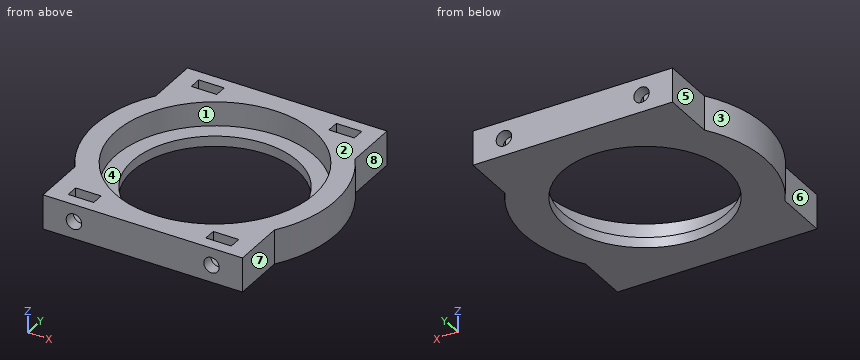
from build123d import *

# Parameters (mm, degrees)
CROQUIS1_R              = 28.9
SALIENTE_EXTRUIR1_DEPTH = 5
CROQUIS2_R              = 28.9
CROQUIS2_R_2            = 24
SALIENTE_EXTRUIR2_DEPTH = 3
CORTAR_EXTRUIR1_DEPTH   = 3.6
CROQUIS6_R              = 2.25
CORTAR_EXTRUIR2_DEPTH   = 10


with BuildPart() as part:
    # Croquis1 → Saliente-Extruir1 (new, symmetric)
    with BuildSketch(Plane.XY):
        with BuildLine():
            Line((-29, 19.595917942), (-29, 35))
            Line((-29, 35), (29, 35))
            Line((29, 35), (29, 19.595917942))
            ThreePointArc((29, 19.595917942), (35, 0), (29, -19.595917942))
            Line((29, -19.595917942), (29, -35))
            Line((29, -35), (-29, -35))
            Line((-29, -35), (-29, -19.595917942))
            ThreePointArc((-29, -19.595917942), (-35, 0), (-29, 19.595917942))
        make_face()
        Circle(CROQUIS1_R, mode=Mode.SUBTRACT)
    extrude(amount=SALIENTE_EXTRUIR1_DEPTH, both=True)

    # Croquis2 → Saliente-Extruir2 (add)
    with BuildSketch(Plane(origin=(0, 0, -5), x_dir=(-1, 0, 0), z_dir=(0, 0, -1))):
        Circle(CROQUIS2_R)
        Circle(CROQUIS2_R_2, mode=Mode.SUBTRACT)
    extrude(amount=-SALIENTE_EXTRUIR2_DEPTH)

    # Croquis5 → Cortar-Extruir1 (cut)
    with BuildSketch(Plane(origin=(0, 28, 0), x_dir=(1, 0, 0), z_dir=(0, 1, 0))):
        Polygon((-23.7, -2.136195996), (-23.7, -5), (-16.3, -5), (-16.3, -2.136195996), (-16.3, 2.136195996), (-20, 4.272391992), (-23.7, 2.136195996), align=None)
        Polygon((16.3, 2.136195996), (16.3, -2.136195996), (16.3, -5), (23.7, -5), (23.7, -2.136195996), (23.7, 2.136195996), (20, 4.272391992), align=None)
    cortar_extruir1 = extrude(amount=CORTAR_EXTRUIR1_DEPTH, mode=Mode.SUBTRACT)

    # Croquis6 → Cortar-Extruir2 (cut)
    with BuildSketch(Plane(origin=(0, 35, 0), x_dir=(1, 0, 0), z_dir=(0, 1, 0))):
        with Locations(Location((-20, 0, 0), (0, 0, 270))):
            Circle(CROQUIS6_R)
        with Locations(Location((20, 0, 0), (0, 0, 270))):
            Circle(CROQUIS6_R)
    cortar_extruir2 = extrude(amount=-CORTAR_EXTRUIR2_DEPTH, mode=Mode.SUBTRACT)

    # Simetría1: Cortar-Extruir1, Cortar-Extruir2 across plane
    add(cortar_extruir1.mirror(Plane.ZX), mode=Mode.SUBTRACT)
    add(cortar_extruir2.mirror(Plane.ZX), mode=Mode.SUBTRACT)


solid = part.part
Check sheet for the modelled part. Datum: model origin and axes. Units: mm. Face numbers are marked on the shaded views. A direction names the side the tool comes from. Give positions to 0.01 mm unless a question says otherwise; leave off trailing zeros. Loops run counter-clockwise (first coordinate to the right, second up) from the corner with the lowest first, then second, coordinate; pieces in that order, holes last. Notation, with made-up numbers: M 19.25,85.25 L 49.25,85.25 A24 ccw 49.25,100.25 Z; hole C 68.5,-20.75 d10. An arc over 180 degrees is marked long. Use a Markdown table: item, result. Add a question column.
Q1. Sectioned sample at C-C, the plane z = -3.25. Record the cut outline in (x, y), then the cut area to 3 significant figures.
Q2. Sectioned sample at A-A, the plane y = 0. Record the cut outline in (x, z).
Q3. Go/stop test with flat-tipped pins: pin 1 (3 mm diameter, centred on y = -30.5, z = 0.5, fed in from +X); pin 2 (4 mm diameter, centred on x = 20, z = 0, fed in from +Y); pin 3 (1.1 mm diameter, centred on y = -30.5, z = 2, fed in from -X); pin 4 (8 mm diameter, centred on x = 7.5, y = 16.5, fed in from -Z). Record where each tip stops, or that it passes through.
Q4. Tool access check on the marked faces 5, 6, 7 and 8. Record the directions out of +Z, -Z, +X, -X, +Y, -Y that give a thin tool (end or side, any length) a straight path to the whole face; none if there is none.
Q5. Mould release check, pull along Y, two halves, no side actions. Record for the marked faces 1, 2, 3 and 4: pulls with the +Y half, pulls with the -Y half, needs draft (parallel to the pull), parting line crosses it, or undercut.
Q6. Scan lines: line 1 along X through (y, z) = (-0.5, 1.75); line 2 along Z through (x, y) = (-20, -27). Record each from-to range of solid material in increasing order. Write a range as [from, to].
Verdict:
| question | item | result |
|---|---|---|
| 1 | outline | M -29,-35 L 29,-35 L 29,-19.6 A35 ccw 29,19.6 L 29,35 L -29,35 L -29,19.6 A35 ccw -29,-19.6 Z; hole C 0,0 d48; hole M -21.77,-31.6 L -18.23,-31.6 L -18.23,-28 L -21.77,-28 Z; hole M -21.77,28 L -18.23,28 L -18.23,31.6 L -21.77,31.6 Z; hole M 18.23,-31.6 L 21.77,-31.6 L 21.77,-28 L 18.23,-28 Z; hole M 18.23,28 L 21.77,28 L 21.77,31.6 L 18.23,31.6 Z |
| 1 | area | 2,520 mm^2 |
| 2 | outline | M -35,-5 L -24,-5 L -24,-2 L -28.9,-2 L -28.9,5 L -35,5 Z; M 24,-5 L 35,-5 L 35,5 L 28.9,5 L 28.9,-2 L 24,-2 Z |
| 3 | pin 1 | x = 29 |
| 3 | pin 2 | y = 25 |
| 3 | pin 3 | x = -29 |
| 3 | pin 4 | through |
| 4 | face 5 | +Z, -Z, -X, +Y |
| 4 | face 6 | +Z, -Z, -X, -Y |
| 4 | face 7 | +Z, -Z, +X, -Y |
| 4 | face 8 | +Z, -Z, +X, +Y |
| 5 | face 1 | undercut |
| 5 | face 2 | needs draft |
| 5 | face 3 | parting line crosses it |
| 5 | face 4 | undercut |
| 6 | line 1 | [-35, -28.9], [28.9, 35] |
| 6 | line 2 | [-5, -2.25], [2.25, 5] |
